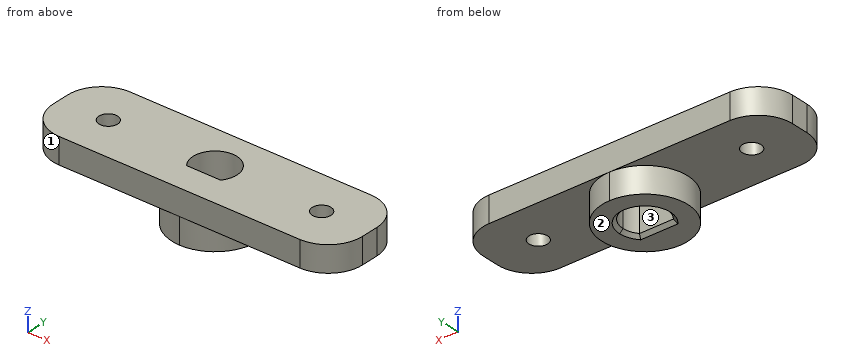
```python
from build123d import *

# Parameters (mm, degrees)
F0_W     = 45.72
F0_H     = 12.7
F0_R     = 1.3843
F1_DEPTH = 3.81
F2_R     = 5.08
F4_DEPTH = 3.81
F5_DEPTH = 12.7
F6_SIZE  = 0.508


with BuildPart() as f1:
    # F0 (on Top) → F1 (new body)
    with BuildSketch(Plane.XY):
        with Locations((0, 6.35)):
            Rectangle(F0_W, F0_H)
        with Locations((-15.76197, 6.35)):
            Circle(F0_R, mode=Mode.SUBTRACT)
        with BuildLine():
            ThreePointArc((-2.511391, 4.3053), (-1.085067, 9.401313), (3.2385, 6.35))
            ThreePointArc((3.2385, 6.35), (3.051313, 5.264933), (2.511391, 4.3053))
            ThreePointArc((2.511391, 4.3053), (0, 3.1115), (-2.511391, 4.3053))
        make_face(mode=Mode.SUBTRACT)
        with Locations((15.76197, 6.35)):
            Circle(F0_R, mode=Mode.SUBTRACT)
        with BuildLine():
            Line((2.511391, 4.3053), (-2.511391, 4.3053))
            ThreePointArc((-2.511391, 4.3053), (0, 3.1115), (2.511391, 4.3053))
        make_face()
        with BuildLine():
            ThreePointArc((2.511391, 4.3053), (3.051313, 5.264933), (3.2385, 6.35))
            ThreePointArc((3.2385, 6.35), (-1.085067, 9.401313), (-2.511391, 4.3053))
            Line((-2.511391, 4.3053), (2.511391, 4.3053))
        make_face()
    extrude(amount=F1_DEPTH)

    # F2
    f2_edges = [f1.edges().sort_by_distance(p)[0] for p in [
        (-22.86, 12.7, 1.905),
        (-22.86, 0, 1.905),
        (22.86, 12.7, 1.905),
        (22.86, 0, 1.905),
    ]]
    fillet(f2_edges, radius=F2_R)

    # F3 (on face) → F4 (join)
    with BuildSketch(Plane(origin=(0, 0, 0), x_dir=(1, 0, 0), z_dir=(0, 0, -1))):
        with BuildLine():
            ThreePointArc((0, -12.7), (4.490128, -10.840128), (6.35, -6.35))
            ThreePointArc((6.35, -6.35), (4.490128, -1.859872), (0, 0))
            ThreePointArc((0, 0), (-6.35, -6.35), (0, -12.7))
        make_face()
    extrude(amount=F4_DEPTH)

    # F0 (on Top) → F5 (cut, symmetric)
    with BuildSketch(Plane.XY):
        with BuildLine():
            ThreePointArc((2.511391, 4.3053), (3.051313, 5.264933), (3.2385, 6.35))
            ThreePointArc((3.2385, 6.35), (-1.085067, 9.401313), (-2.511391, 4.3053))
            Line((-2.511391, 4.3053), (2.511391, 4.3053))
        make_face()
    extrude(amount=F5_DEPTH, both=True, mode=Mode.SUBTRACT)

    # F6
    f6_edges = [f1.edges().sort_by_distance(p)[0] for p in [
        (0, 4.3053, -3.81),
        (0, 9.5885, -3.81),
    ]]
    chamfer(f6_edges, length=F6_SIZE)


solid = f1.part
```
Could you check a few things on this model? Use its own coordinates, in mm. Face numbers are marked on the shaded views. Give positions to 0.01 mm unless a question says otherwise; leave off trailing zeros. Loops run counter-clockwise (first coordinate to the right, second up) from the corner with the lowest first, then second, coordinate; pieces in that order, holes last. Notation, with made-up numbers: (-11.75, 0.25) - (27.25, 0.25) arc R26 cw to (27.25, 21.25) - close; hole circle Ø5 at (-38.75, 56). An arc over 180 degrees is marked (long way). Answer in a Markdown table with one row per item. Add a question column.
Q1. If we section it at B-B (x = 16): List the corners of the cut face in (y, z) for me, plus the area to 3 significant figures.
Q2. We'd pull the mould along X, two halves only. Please class the marked faces 1, 2 and 3: +X half, -X half, draft (parallel to the pull), parting line (faces both ways), or undercut.
Q3. Please list where these lines run through material, in increasing order: L1, parallel to Y at x = 0, z = 2.5; L2, parallel to Z at x = -7.5, y = 0.5; L3, parallel to X at y = 5, z = -0.5. Write a range as from..to.
Q4. If we section it at C-C (z = -1.5): List the corners of the cut face in (x, y) for me.
Q5. For pin 1 (6.5 mm diameter, centred on x = -16, y = 9.5, fed in from -Z), with a flat end and sliding along its axis, tell me the tip position at first contact or that it passes through.
Q6. If we section it at D-D (y = 5.75): State how many separate pieces and enclosed holes the cut face has, plus the area to 3 significant figures.
Q7. If we section it at A-A (z = 1.25): List the corners of the cut face in (x, y) for me.
The answers:
| question | item | result |
|---|---|---|
| 1 | outline | (0, 0) - (4.99, 0) - (4.99, 3.81) - (0, 3.81) - close; (7.71, 0) - (12.7, 0) - (12.7, 3.81) - (7.71, 3.81) - close |
| 1 | area | 38.0 mm^2 |
| 2 | face 1 | -X half |
| 2 | face 2 | draft |
| 2 | face 3 | undercut |
| 3 | L1 | y = 0..4.31, 9.59..12.7 |
| 3 | L2 | z = 0..3.81 |
| 3 | L3 | x = -6.2..-2.94, 2.94..6.2 |
| 4 | outline | circle Ø12.7 at (0, 6.35); hole (-2.51, 4.31) - (2.51, 4.31) arc R3.24 ccw to (3.24, 6.35) arc R3.24 ccw (long way) to start |
| 5 | pin 1 | stops at z = 0 |
| 6 | separate pieces | 4 |
| 6 | enclosed holes | 0 |
| 6 | area | 155 mm^2 |
| 7 | outline | (-22.86, 5.08) arc R5.08 ccw to (-17.78, 0) - (17.78, 0) arc R5.08 ccw to (22.86, 5.08) - (22.86, 7.62) arc R5.08 ccw to (17.78, 12.7) - (-17.78, 12.7) arc R5.08 ccw to (-22.86, 7.62) - close; hole circle Ø2.77 at (-15.76, 6.35); hole (-2.51, 4.31) - (2.51, 4.31) arc R3.24 ccw to (3.24, 6.35) arc R3.24 ccw (long way) to start; hole circle Ø2.77 at (15.76, 6.35) |
